CAD build for the part. Positions are in the model's coordinates, mm. A direction names the side the tool comes from. Round coordinates to 2 decimals unless told otherwise and drop trailing zeros. Order: outer loops, then holes, each group sorted by start corner. A loop starts at its lowest first (then second) coordinate and runs counter-clockwise, first axis right, second up. Notation, with made-up numbers: (-12.5, 6.25) -> (5.5, 6.25) arc R21 cw to (5.5, 25.25) -> close; hole circle Ø6 at (57.25, 67.25). An arc over 180 degrees is marked (long way). Return JSON: item names as keys, results as strings. Group by question number.
Q1. Cut at B-B (x = -6.5). Write the cut outline in (y, z), then the cut area to 4 significant figures.
Q2. Cut at D-D (y = -8.5). Write the cut outline in (x, z).
Q3. Flat gauge pins, fed straight in: pin 1 (1.4 mm diameter, centred on x = -9.5, y = -8.5, fed in from -Z); pin 2 (0.8 mm diameter, centred on x = -16, z = 0, fed in from -Y); pin 3 (4 mm diameter, centred on x = -5.5, z = -2, fed in from -Y). Where does each tip first touch, or does it go through?
Q4. Cut at C-C (y = 1.5). Write the cut outline in (x, z), then the cut area to 3 significant figures.
Q5. Cut at A-A (z = -0.5). Write the cut outline in (x, y), then the cut area to 3 significant figures.
Q6. Probe line 1 along X through (y, z) = (-4, -2); line 2 along Y through (x, z) = (1, 1.25); line 3 along Z through (x, y) = (15.5, -1.25). List the from-to ranges inside material, lowest first.
Q7. Which spindle directions (+Z, -Z, +X, -X, +Y, -Y) get a long thin tool onto all of the face, cutting with end or side? Do faces 1 (the flat face through (-8, -9, -2.25)), 2 (the flat face through (-8, -9, 2.25)), 3 (the flat face through (-16, 0, -2)). Say none if no direction does.
from build123d import *

# Parameters (mm, degrees)
SKETCH_1_W      = 30
SKETCH_1_H      = 15
EXTRUDE_1_DEPTH = 3.75
SKETCH_2_W      = 4
SKETCH_2_H      = 4
EXTRUDE_2_DEPTH = 2.5
EXTRUDE_3_DEPTH = 2.25
FILLET_1_R      = 1


with BuildPart() as part:
    # 草图1 → 凸台-拉伸1 (new, symmetric)
    with BuildSketch(Plane.XY):
        Rectangle(SKETCH_1_W, SKETCH_1_H)
    extrude(amount=EXTRUDE_1_DEPTH, both=True)

    # 草图2 → 凸台-拉伸2 (add)
    with BuildSketch(Plane.ZY.offset(15)):
        Rectangle(SKETCH_2_W, SKETCH_2_H)
    extrude_2 = extrude(amount=EXTRUDE_2_DEPTH)

    # 镜向1: 凸台-拉伸2 across plane
    add(extrude_2.mirror(Plane(origin=(0, 0, 0), x_dir=(0, 0, 1), z_dir=(1, 0, 0))))

    # 草图4 → 凸台-拉伸3 (add, symmetric)
    with BuildSketch(Plane.XY):
        Polygon((-12.5, -7.5), (-8, -10.5), (-3.5, -7.5), align=None)
    extrude(amount=EXTRUDE_3_DEPTH, both=True)

    # 圆角1
    fillet_1_edges = [part.edges().sort_by_distance(p)[0] for p in [
        (-8, -10.5, 0),
    ]]
    fillet(fillet_1_edges, radius=FILLET_1_R)


solid = part.part
Solution:
{
 "1": {"outline": "(-9.5, -2.25) -> (-7.5, -2.25) -> (-7.5, -3.75) -> (7.5, -3.75) -> (7.5, 3.75) -> (-7.5, 3.75) -> (-7.5, 2.25) -> (-9.5, 2.25) -> close", "area": "121.5 mm²"},
 "2": {"outline": "(-11, -2.25) -> (-5, -2.25) -> (-5, 2.25) -> (-11, 2.25) -> close"},
 "3": {"pin 1": "stops at z = -2.25", "pin 2": "stops at y = -2", "pin 3": "stops at y = -10.16"},
 "4": {"outline": "(-17.5, -2) -> (-15, -2) -> (-15, -3.75) -> (15, -3.75) -> (15, -2) -> (17.5, -2) -> (17.5, 2) -> (15, 2) -> (15, 3.75) -> (-15, 3.75) -> (-15, 2) -> (-17.5, 2) -> close", "area": "245 mm²"},
 "5": {"outline": "(-17.5, -2) -> (-15, -2) -> (-15, -7.5) -> (-12.5, -7.5) -> (-8.55, -10.13) arc R1 ccw to (-7.45, -10.13) -> (-3.5, -7.5) -> (15, -7.5) -> (15, -2) -> (17.5, -2) -> (17.5, 2) -> (15, 2) -> (15, 7.5) -> (-15, 7.5) -> (-15, 2) -> (-17.5, 2) -> close", "area": "483 mm²"},
 "6": {"line 1": "x = -15 to 15", "line 2": "y = -7.5 to 7.5", "line 3": "z = -2 to 2"},
 "7": {"face 1": "-Z, +X, -X, -Y", "face 2": "+Z, +X, -X, -Y", "face 3": "-Z, -X, +Y, -Y"}
}
